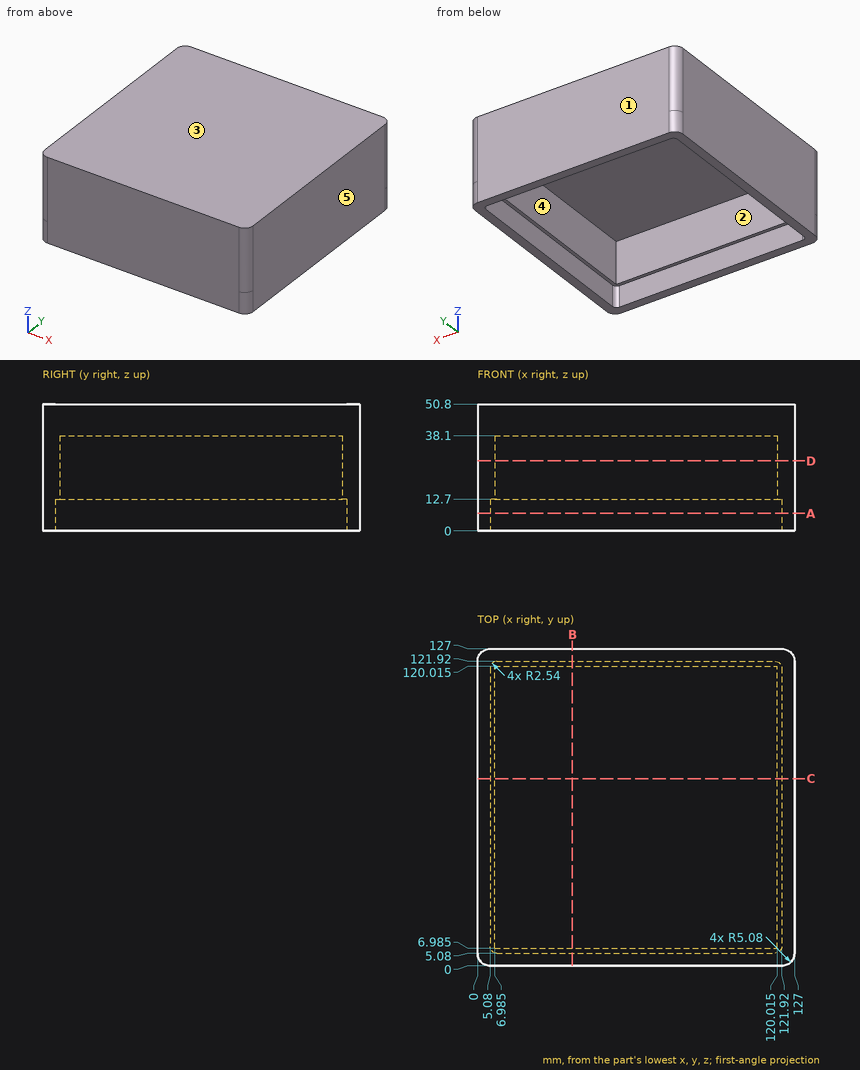
Source: three-view drawing plus pictorial views. Frame: mm from the lowest corner of the part. A direction names the side the tool comes from. Coordinates: 2 decimals unless noted, no trailing zeros. Loops run counter-clockwise (first coordinate to the right, second up) from the corner with the lowest first, then second, coordinate; pieces in that order, holes last. Notation, with made-up numbers: (58, -14) -> (78, -14) arc R15 ccw to (78, 1) -> close; hole circle Ø10 at (-14, 5.5). An arc over 180 degrees is marked (long way). Answer in a Markdown table with one row per item. Add a question column.
Q1. Pull-direction query (X, two-part tool) for the marked faces 3, 4 and 5; classes: pulls with the +X half, pulls with the -X half, needs draft (parallel to the pull), parting line crosses it, or undercut.
Q2. Ray query, line 1 along Y through (x, z) = (21.5, 38) (3 decimals); line 2 along X through (y, z) = (101, 8). Return the intervals inside material, ascending.
Q3. Section D-D on z = 28. Return the cut outline in (x, y) (3 decimals), and give its area (3 significant figures).
Q4. Reachability of the marked faces 1 and 2 from +Z, -Z, +X, -X, +Y, -Y: full face, straight path, thin tool, end or side. Return the list, or none.
Q5. Section A-A on z = 7. Return the cut outline in (x, y).
Q6. Section B-B on x = 38. Return the cut outline in (y, z) (3 decimals).
Q7. Contact query for a flat-ended pin moving along its axis: pin 1 Ø1 at (x, y) = (88, 113) entering from -Z. Output: stop coordinate, or through.
Computed values:
| question | item | result |
|---|---|---|
| 1 | face 3 | needs draft |
| 1 | face 4 | undercut |
| 1 | face 5 | pulls with the +X half |
| 2 | line 1 | y = 0 to 6.985, 120.015 to 127 |
| 2 | line 2 | x = 0 to 5.08, 121.92 to 127 |
| 3 | outline | (0, 5.08) arc R5.08 ccw to (5.08, 0) -> (121.92, 0) arc R5.08 ccw to (127, 5.08) -> (127, 121.92) arc R5.08 ccw to (121.92, 127) -> (5.08, 127) arc R5.08 ccw to (0, 121.92) -> close; hole (6.985, 6.985) -> (120.015, 6.985) -> (120.015, 120.015) -> (6.985, 120.015) -> close |
| 3 | area | 3,330 mm^2 |
| 4 | face 1 | +Z, -Z, +X, -X, +Y |
| 4 | face 2 | -Z |
| 5 | outline | (0, 5.08) arc R5.08 ccw to (5.08, 0) -> (121.92, 0) arc R5.08 ccw to (127, 5.08) -> (127, 121.92) arc R5.08 ccw to (121.92, 127) -> (5.08, 127) arc R5.08 ccw to (0, 121.92) -> close; hole (5.08, 7.62) arc R2.54 ccw to (7.62, 5.08) -> (119.38, 5.08) arc R2.54 ccw to (121.92, 7.62) -> (121.92, 119.38) arc R2.54 ccw to (119.38, 121.92) -> (7.62, 121.92) arc R2.54 ccw to (5.08, 119.38) -> close |
| 6 | outline | (0, 0) -> (5.08, 0) -> (5.08, 12.7) -> (6.985, 12.7) -> (6.985, 38.1) -> (120.015, 38.1) -> (120.015, 12.7) -> (121.92, 12.7) -> (121.92, 0) -> (127, 0) -> (127, 50.8) -> (0, 50.8) -> close |
| 7 | pin 1 | stops at z = 38.1 |
